```python
from build123d import *

# Parameters (mm, degrees)
F0_R          = 4
F0_R_2        = 3
F1_DEPTH      = 7.5
F1_DEPTH_BACK = 12.5
F0_R_3        = 4.5
F2_DEPTH      = 12.5
F3_W          = 12
F3_H          = 9.086956
F4_DEPTH      = 25
F4_DEPTH_BACK = 25


with BuildPart() as f1:
    # F0 (on Right) → F1 (new body, two sides)
    with BuildSketch(Plane.YZ) as f1_sk:
        Circle(F0_R)
        Circle(F0_R_2, mode=Mode.SUBTRACT)
    extrude(amount=F1_DEPTH)
    extrude(f1_sk.sketch, amount=-F1_DEPTH_BACK)

    # F0 (on Right) → F2 (join)
    with BuildSketch(Plane.YZ):
        Circle(F0_R_3)
        Circle(F0_R, mode=Mode.SUBTRACT)
    extrude(amount=-F2_DEPTH)

    # F3 (on Front) → F4 (cut, two sides)
    with BuildSketch(Plane.XZ) as f4_sk:
        with Locations((-5.5, 6.543478)):
            Rectangle(F3_W, F3_H)
    extrude(amount=F4_DEPTH, mode=Mode.SUBTRACT)
    extrude(f4_sk.sketch, amount=-F4_DEPTH_BACK, mode=Mode.SUBTRACT)


solid = f1.part
```
Can you work these out from the model? Positions are in its coordinate system, mm. A direction names the side the tool comes from. Coordinates: 2 decimals unless noted, no trailing zeros. Loops run counter-clockwise (first coordinate to the right, second up) from the corner with the lowest first, then second, coordinate; pieces in that order, holes last. Notation, with made-up numbers: (-18, 70) -> (28, 70) arc R20 cw to (28, 96) -> close; hole circle Ø5 at (4.5, 44). An arc over 180 degrees is marked (long way). Put each result on its own line as item: value. Start each with the question number.
Q1. If I drill on line 1 (Z direction, x = 3, y = 0); line 2 (Y direction, x = 5.25, z = -2); line 3 (Z direction, x = -8.5, y = 0), over which ranges is the centre line in solid material (lowest first)? Write a range as [from, to].
Q2. For faces 5 (the face through (3.802, -0.867, -3.905)), 6 (the face through (7.5, 1, 3)), 7 (the face through (0.5, 0, 3.2)), which set-ups out of +Z, -Z, +X, -X, +Y, -Y let a thin tool reach every point of the face, with its end or its side?
Q3. I want a section at A-A (y = 0). Write out the boundary of the cut face in (x, z), plus the area to 4 significant figures.
Q4. I'm going to push flat-ended pins straight in: P1, Ø2, axis at x = -4, y = -1, coming from the +Z side; P2, Ø1.4, axis at x = -7.5, y = 3, coming from the +Z side. Where does each tip first touch, or does it pass through?
Q5. I want a section at B-B (z = -2). Write out the boundary of the cut face in (x, y).
Q6. I want a section at D-D (x = 6.25). Write out the boundary of the cut face in (y, z).
Q7. Thinking about a two-plate mould opening in X: for faces 1 (the face through (-6, -3, 2)), 2 (the face through (-12.5, 1, -3)), 3 (the face through (-6, 3, 2)), 4 (the face through (0, -0.7, -4.1)), which applies, pulls with the +X half, pulls with the -X half, needs draft (parallel to the pull), parting line crosses it, or undercut?
Q8. I want a section at C-C (y = -2.5). Write out the boundary of the cut face in (x, z), plus the area to 3 significant figures.
Taken from the geometry:
1. line 1: z = [-4, -3], [3, 4]
1. line 2: y = [-3.46, -2.24], [2.24, 3.46]
1. line 3: z = [-4.5, -3]
2. face 5: +X
2. face 6: +Z, -Z, +X, +Y, -Y
2. face 7: +Z, +Y, -Y
3. outline: (-12.5, -4.5) -> (0, -4.5) -> (0, -4) -> (7.5, -4) -> (7.5, -3) -> (-12.5, -3) -> close; (-12.5, 3) -> (-11.5, 3) -> (-11.5, 4.5) -> (-12.5, 4.5) -> close; (0.5, 3) -> (7.5, 3) -> (7.5, 4) -> (0.5, 4) -> close
3. area: 34.75 mm2
4. P1: stops at z = -2.24
4. P2: stops at z = 2
5. outline: (-12.5, -4.03) -> (0, -4.03) -> (0, -3.46) -> (7.5, -3.46) -> (7.5, -2.24) -> (-12.5, -2.24) -> close; (-12.5, 2.24) -> (7.5, 2.24) -> (7.5, 3.46) -> (0, 3.46) -> (0, 4.03) -> (-12.5, 4.03) -> close
6. outline: circle Ø8 at (0, 0); hole circle Ø6 at (0, 0)
7. face 1: undercut
7. face 2: pulls with the -X half
7. face 3: undercut
7. face 4: pulls with the +X half
8. outline: (-12.5, -3.74) -> (0, -3.74) -> (0, -3.12) -> (7.5, -3.12) -> (7.5, -1.66) -> (-12.5, -1.66) -> close; (-12.5, 1.66) -> (7.5, 1.66) -> (7.5, 3.12) -> (0.5, 3.12) -> (0.5, 2) -> (-11.5, 2) -> (-11.5, 3.74) -> (-12.5, 3.74) -> close
8. area: 53.5 mm2
